Autodesk Fusion 360 part; units mm, degrees
sketch "Sketch1" plane through (0, 0, 0) normal (0, 0, 1) x (1, 0, 0)
  circle A0 centre (0, 0) radius 23
  circle A1 centre (0, 0) radius 24.5
  dimension "d1" = 46
  dimension "d2" = 49
extrude "Extrude1" add sketch "Sketch1" along normal blind 12
sketch "Sketch2" plane through (0, 0, 12) normal (0, 0, 1) x (-1, 0, 0)
  circle A0 centre (0, 0) radius 23
  circle A1 centre (0, 0) radius 24.5
  circle A2 centre (0, 0) radius 2
  circle A3 centre (0, 0) radius 24.5
  dimension "d5" = 4
extrude "Extrude2" add sketch "Sketch2" along normal blind 3 contours A0 | A1 A3
fillet "Fillet1" radius 4 1 edges at (22.842, 8.8596, 15)
sketch "Sketch3" plane through (0, 0, 0) normal (0, 1, 0) x (1, 0, 0)
  line L0 (0, 0) -> (0, -4.5)
  circle A0 centre (0, -4.5) radius 2
  dimension "d10" = 4.5
  dimension "d11" = 4
extrude "Extrude3" cut sketch "Sketch3" along normal mid plane 700
fillet "Fillet2" radius 0.75 2 edges at (-22.842, -8.8596, 0) (-21.4435, 8.3172, 0)
Part model, mm, in its own coordinate system. A direction names the side the tool comes from. Coordinates: 2 decimals unless noted, no trailing zeros. Order: outer loops, then holes, each group sorted by start corner. A loop starts at its lowest first (then second) coordinate and runs counter-clockwise, first axis right, second up. Notation, with made-up numbers: (56.5, 29) -> (86.5, 29) arc R26 ccw to (86.5, 57) -> close; hole circle Ø7 at (40, 20). An arc over 180 degrees is marked (long way). Put each result on its own line as item: value. Start each with the question number.
(1) Band-saw the part on A-A (x = 0). Count the separate pieces of the cut face and the enclosed holes in it, then the cut area to 3 significant figures.
(2) Probe line 1 along Y through (x, z) = (0, 1.25); line 2 along Z through (x, y) = (0, 23.5); line 3 along Y through (x, z) = (9.5, 1.25). List the from-to ranges inside material, lowest first. Write a range as [from, to].
(3) Pin check, flat tips, straight feed: pin 1 Ø3 at (x, z) = (-5, 12.5) entering from -Y; pin 2 Ø4 at (y, z) = (-10, 10.5) entering from -X; pin 3 Ø1 at (y, z) = (6.5, 6) entering from -X. Stop position of each tip, or through.
(4) Which spindle directions (+Z, -Z, +X, -X, +Y, -Y) get a long thin tool onto all of the face, cutting with end or side? Do faces 1 (the face through (1.847, 23.695, 3.734)), 2 (the face through (0, 5, 12)). Say none if no direction does.
(5) Mould opens along Y. For faces 3 (the face through (0, 4, 15)), 4 (the face through (13.17, -20.66, 5.8)), 5 (the face through (0, -2, 13)) say: pulls with the +Y half, pulls with the -Y half, needs draft (parallel to the pull), parting line crosses it, or undercut.
(6) Band-saw the part on D-D (z = 13.5). Give the cut face in (x, y) (1 decimal).
Determined:
1. separate pieces: 4
1. enclosed holes: 0
1. area: 152 mm²
2. line 1: y = [-24.5, -23], [23, 24.5]
2. line 2: z = [0.04, 2.5], [6.5, 13.65]
2. line 3: y = [-22.58, -20.95], [20.95, 22.58]
3. pin 1: stops at y = -24.16
3. pin 2: stops at x = -23.16
3. pin 3: stops at x = -23.75
4. face 1: +Y, -Y
4. face 2: -Z
5. face 3: needs draft
5. face 4: parting line crosses it
5. face 5: undercut
6. outline: circle Ø47.2 at (0, 0); hole circle Ø4 at (0, 0)
